from build123d import *

# Parameters (mm, degrees)
SKETCH_1_W          = 8
SKETCH_1_H          = 8
SKETCH_1_W_2        = 3.05
SKETCH_1_H_2        = 3.05
EXTRUDE_1_DEPTH     = 7.5
SKETCH_2_W          = 8
SKETCH_2_H          = 8
EXTRUDE_2_DEPTH     = 0.5
EXTRUDE_3_DEPTH     = 8
SKETCH_4_R          = 0.95
EXTRUDE_4_DEPTH     = 4
SKETCH_4_2_R        = 0.95
CUT_EXTRUDE_1_DEPTH = 4.2


with BuildPart() as part:
    # 草图1 → 凸台-拉伸1 (new body)
    with BuildSketch(Plane(origin=(0, 0, 0), x_dir=(1, 0, 0), z_dir=(0, 1, 0))):
        with Locations((4, 4)):
            Rectangle(SKETCH_1_W, SKETCH_1_H)
        with Locations((4, 4)):
            Rectangle(SKETCH_1_W_2, SKETCH_1_H_2, mode=Mode.SUBTRACT)
    extrude(amount=EXTRUDE_1_DEPTH)

    # 草图2 → 凸台-拉伸2 (add)
    with BuildSketch(Plane(origin=(0, 7.5, 0), x_dir=(1, 0, 0), z_dir=(0, 1, 0))):
        with Locations((4, 4)):
            Rectangle(SKETCH_2_W, SKETCH_2_H)
    extrude(amount=EXTRUDE_2_DEPTH)

    # 草图3 → 凸台-拉伸3 (add)
    with BuildSketch(Plane(origin=(8, 0, 0), x_dir=(0, 0, -1), z_dir=(1, 0, 0))):
        Polygon((12.042467117, 13.849699628), (12.712142643, 10.720556823), (0, 8), (-0.669675526, 11.129142804), align=None)
        Polygon((8, 8), (12.712142643, 10.720556823), (0, 8), align=None)
    extrude(amount=-EXTRUDE_3_DEPTH)

    # 草图4 → 凸台-拉伸4 (add)
    with BuildSketch(Plane(origin=(0, 10.778779281, 2.306792989), x_dir=(1, 0, 0), z_dir=(0, 0.9778571263703284, 0.2092736017914434))):
        with Locations((4, 3.924188814)):
            Circle(SKETCH_4_R)
        with Locations((4, 12.424188814)):
            Circle(SKETCH_4_R)
    extrude(amount=-EXTRUDE_4_DEPTH)

    # 草图4<2> → 切除-拉伸1 (cut)
    with BuildSketch(Plane(origin=(0, 10.778779281, 2.306792989), x_dir=(1, 0, 0), z_dir=(0, 0.9778571263703284, 0.2092736017914434))):
        with Locations(Location((4, 3.924188814, 0), (0, 0, 270))):
            Circle(SKETCH_4_2_R)
        with Locations(Location((4, 12.424188814, 0), (0, 0, 242.456788252))):
            Circle(SKETCH_4_2_R)
    extrude(amount=-CUT_EXTRUDE_1_DEPTH, mode=Mode.SUBTRACT)


solid = part.part
Input: part model. Units: mm. Frame: model coordinates. A direction names the side the tool comes from. Give positions to 0.01 mm unless a question says otherwise; leave off trailing zeros. Order: outer loops, then holes, each group sorted by start corner. A loop starts at its lowest first (then second) coordinate and runs counter-clockwise, first axis right, second up. Notation, with made-up numbers: (8.25, -14) -> (15.25, -14) arc R23 cw to (15.25, 8) -> close; hole circle Ø3 at (-1, 29.25). An arc over 180 degrees is marked (long way). Use one line per item in the form item = value.
1) Section A-A, the plane y = 6.25. Return loops of the section in (x, z) (3 decimals).
Response values:
outline = (0, -8) -> (8, -8) -> (8, 0) -> (0, 0) -> close; hole (2.475, -5.525) -> (5.525, -5.525) -> (5.525, -2.475) -> (2.475, -2.475) -> close
2) Reachability of faces 4 (the flat face through (4.013, 7.452, -2.216)), 5 (the flat face through (4, 4, -5.525)), 6 (the flat face through (4, 4, -8)), 7 (the flat face through (6, 0, -4)), 8 (the flat face through (4, 4, 0)) from +Z, -Z, +X, -X, +Y, -Y: full face, straight path, thin tool, end or side. Return the list, or none.
Response values:
face_4 = none
face_5 = -Y
face_6 = -Z, +X, -X, -Y
face_7 = +Z, -Z, +X, -X, -Y
face_8 = +Z, +X, -X, -Y
3) Section B-B, the plane x = 7.25. Return loops of the section in (y, z), and give its area (3 significant figures).
Response values:
outline = (0, -8) -> (8, -8) -> (10.72, -12.71) -> (13.85, -12.04) -> (11.13, 0.67) -> (8, 0) -> (0, 0) -> close
area = 116 mm^2
4) Line query: probe 1 along Z at (x, y) = (5, 5.5) (3 decimals); probe 2 along X at (y, z) = (5, -4) (3 decimals); probe 3 along Z at (x, y) = (4, 9.5). Output: solid intervals per line, ascending.
Response values:
probe_1 = -8 to -5.525, -2.475 to 0
probe_2 = 0 to 2.475, 5.525 to 8
probe_3 = -9.7 to -2.95, -1.01 to 0.32
5) Section D-D, the plane z = -6.5. Return loops of the section in (x, y), and give its area (3 significant figures).
Response values:
outline = (0, 0) -> (8, 0) -> (8, 12.66) -> (0, 12.66) -> close
area = 101 mm^2
6) First-contact query: pin 1 Ø1 at (x, z) = (4, -6) entering from +Y; pin 2 Ø1.5 at (x, y) = (4.5, 4) entering from +Z; pin 3 Ø4 at (x, y) = (5.5, 4) entering from -Z. Flat tips, straight axial feed; report the tip coordinate or a pass-through.
Response values:
pin_1 = 12.66
pin_2 = 0
pin_3 = -8
7) Mould query, pull axis Y, two halves, no side actions, for faces 1 (the cylindrical face through (4.47, 11.18, -9.47)), 2 (the flat face through (4.06, 9.54, 0.33)), 3 (the flat face through (4, 4, -2.475)). Classes: pulls with the +Y half, pulls with the -Y half, needs draft (parallel to the pull), parting line crosses it, or undercut.
Response values:
face_1 = undercut
face_2 = pulls with the -Y half
face_3 = needs draft
